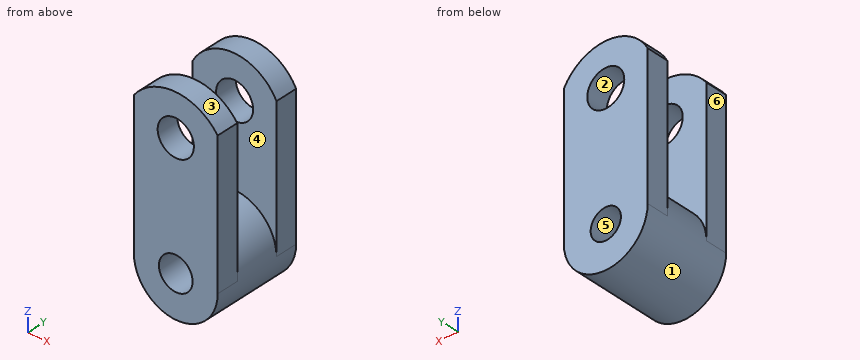
```python
from build123d import *

# Parameters (mm, degrees)
F0_R      = 23.7382132345
F1_DEPTH  = 50.8
F2_R      = 9.5504796537
F3_DEPTH  = 25.4
F4_R      = 8.5638867121
F5_DEPTH  = 25.4
F7_DEPTH  = 12.7
F9_DEPTH  = 12.7
F10_R     = 10.4784811222
F11_DEPTH = 25.4
F12_R     = 10.2578484405
F13_DEPTH = 25.4


with BuildPart() as f1:
    # F0 (on Front) → F1 (new body)
    with BuildSketch(Plane.XZ):
        Circle(F0_R)
    extrude(amount=F1_DEPTH)

    # F2 (on face) → F3 (cut)
    with BuildSketch(Plane.XZ.offset(50.8)):
        Circle(F2_R)
    extrude(amount=-F3_DEPTH, mode=Mode.SUBTRACT)

    # F4 (on face) → F5 (cut)
    with BuildSketch(Plane(origin=(0, 0, 0), x_dir=(-1, 0, 0), z_dir=(0, 1, 0))):
        Circle(F4_R)
    extrude(amount=-F5_DEPTH, mode=Mode.SUBTRACT)

    # F6 (on face) → F7 (join)
    with BuildSketch(Plane.XZ.offset(50.8)):
        with BuildLine():
            Line((-23.7382132345, 80.9877067804), (-23.7382132345, 0))
            ThreePointArc((-23.7382132345, 0), (0, 23.7382132345), (23.7382132345, 0))
            Line((23.7382132345, 0), (23.7382132345, 80.9877067804))
            ThreePointArc((23.7382132345, 80.9877067804), (0, 92.9128323783), (-23.7382132345, 80.9877067804))
        make_face()
    extrude(amount=-F7_DEPTH)

    # F8 (on face) → F9 (join)
    with BuildSketch(Plane(origin=(0, 0, 0), x_dir=(-1, 0, 0), z_dir=(0, 1, 0))):
        with BuildLine():
            Line((-23.7382132345, 79.5382484794), (-23.7382132345, 0))
            ThreePointArc((-23.7382132345, 0), (0, 23.7382132345), (23.7382132345, 0))
            Line((23.7382132345, 0), (23.7382132345, 79.5382484794))
            ThreePointArc((23.7382132345, 79.5382484794), (0, 93.6788109579), (-23.7382132345, 79.5382484794))
        make_face()
    extrude(amount=-F9_DEPTH)

    # F10 (on face) → F11 (cut)
    with BuildSketch(Plane(origin=(0, 0, 0), x_dir=(-1, 0, 0), z_dir=(0, 1, 0))):
        with Locations((0, 69.4402828813)):
            Circle(F10_R)
    extrude(amount=-F11_DEPTH, mode=Mode.SUBTRACT)

    # F12 (on face) → F13 (cut)
    with BuildSketch(Plane.XZ.offset(50.8)):
        with Locations((0, 69.3438276649)):
            Circle(F12_R)
    extrude(amount=-F13_DEPTH, mode=Mode.SUBTRACT)


solid = f1.part
```
For this review, take the finished solid that the model builds, in its own axes (mm). Face numbers are marked on the shaded views. A direction names the side the tool comes from. Give positions to 0.01 mm unless a question says otherwise; leave off trailing zeros. Write each loop counter-clockwise with the first axis right and the second up, starting at its lowest first coordinate (ties: lowest second). Pieces come first, ordered by that corner, then holes. Notation, with made-up numbers: M -34.75,57.25 L 14.25,57.25 A19 cw 14.25,90.25 Z; hole C 4.25,51.5 d1. An arc over 180 degrees is marked long. One line per item, written item: value.
1) Take a section at B-B, the plane z = 49.5. Write out the cut boundary in (x, y).
Results are:
outline: M -23.74,-50.8 L 23.74,-50.8 L 23.74,-38.1 L -23.74,-38.1 Z; M -23.74,-12.7 L 23.74,-12.7 L 23.74,0 L -23.74,0 Z
2) Take a section at C-C, the plane y = -34. Write out the cut boundary in (x, z).
Results are:
outline: C 0,0 d47.48; hole C 0,0 d19.1
3) Take a section at A-A, the plane x = 0. Write out the cut boundary in (y, z), then the cut area to 3 significant figures.
Results are:
outline: M -50.8,-23.74 L 0,-23.74 L 0,-8.56 L -25.4,-8.56 L -25.4,-9.55 L -50.8,-9.55 Z; M -50.8,9.55 L -25.4,9.55 L -25.4,8.56 L 0,8.56 L 0,58.96 L -12.7,58.96 L -12.7,23.74 L -38.1,23.74 L -38.1,59.09 L -50.8,59.09 Z; M -50.8,79.6 L -38.1,79.6 L -38.1,92.91 L -50.8,92.91 Z; M -12.7,79.92 L 0,79.92 L 0,93.68 L -12.7,93.68 Z
area: 2,730 mm²
4) For line 1 (X direction, y = -43.5, z = 70); line 2 (Z direction, x = 0, y = -6.25); line 3 (X direction, y = -11.5, z = 75.5), list the stretches that pass through material, from the lowest coordinate up. Write a range as from..to.
Results are:
line 1: x = -23.74..-10.24, 10.24..23.74
line 2: z = -23.74..-8.56, 8.56..58.96, 79.92..93.68
line 3: x = -23.74..-8.55, 8.55..23.74
5) For P1, Ø10, axis at x = 15.5, y = -40, coming from the -Z side; P2, Ø8, axis at x = 11.5, y = -21, coming from the -Z side; P3, Ø12, axis at x = -8, y = -6, coming from the +Z side; P4, Ø12.5, axis at x = 0, z = 69.34, coming from the +Y side, all flat-tipped, find the tip position at first contact; note any pin that passes through.
Results are:
P1: stops at z = -21.29
P2: stops at z = -22.52
P3: stops at z = 93.6
P4: passes through
6) For the marked faces 1, 2 and 3, list the 3-axis set-ups (+Z, -Z, +X, -X, +Y, -Y) from which the entire face can be reached by the end or side of a thin tool; tool diameter is ignored.
Results are:
face 1: none
face 2: +Y
face 3: +Z, -Y
7) Take a section at D-D, the plane x = 15. Write out the cut boundary in (y, z).
Results are:
outline: M -50.8,-18.4 L 0,-18.4 L 0,89.13 L -12.7,89.13 L -12.7,18.4 L -38.1,18.4 L -38.1,88.83 L -50.8,88.83 Z
8) The part is to be moulded in two halves that separate along X. For the marked faces 4, 5 and 6, say which applies: +X half, -X half, draft (parallel to the pull), parting line (faces both ways), or undercut.
Results are:
face 4: draft
face 5: undercut
face 6: -X half
